```python
from build123d import *

# Parameters (mm, degrees)
BOX006_W        = 88.9
BOX006_H        = 88.9
BOX006_DEPTH    = 2438.4
SKETCH003_W     = 38.1
SKETCH003_H     = 88.9
POCKET003_DEPTH = 88.9010000032
POCKET009_DEPTH = 88.901
POCKET013_DEPTH = 38.1
SKETCH018_W     = 38.1
SKETCH018_H     = 101.6
POCKET015_DEPTH = 88.901


with BuildPart() as obj1:
    # Box006 → Box006 (new body)
    with BuildSketch(Plane(origin=(1435.1, 1435.1, 0), x_dir=(1, 0, 0), z_dir=(0, 0, 1))):
        with Locations((44.45, 44.45)):
            Rectangle(BOX006_W, BOX006_H)
    extrude(amount=BOX006_DEPTH)

    # Sketch003 → Pocket003 (cut, through all)
    with BuildSketch(Plane(origin=(1435.1, 1435.1, 0), x_dir=(1, 0, 0), z_dir=(0, -1, 0))):
        with Locations((69.85, 501.65)):
            Rectangle(SKETCH003_W, SKETCH003_H)
    extrude(amount=-POCKET003_DEPTH, mode=Mode.SUBTRACT)


with BuildPart() as pocket015:
    # Part__Mirroring: instance of obj1
    add(obj1.part.mirror(Plane(origin=(762, 0, 0), x_dir=(0, -1, 0), z_dir=(1, 0, 0))))

    # Sketch010 → Pocket009 (cut, through all)
    with BuildSketch(Plane(origin=(0, 0, 0), x_dir=(0, -1, 0), z_dir=(-1, 0, 0))):
        Polygon((-1524.003048, 2221.9412), (-1524.003048, 2438.4), (-1434.087048, 2438.4), (-1434.087048, 2189.2144524157), align=None)
    extrude(amount=-POCKET009_DEPTH, mode=Mode.SUBTRACT)

    # Sketch014 → Pocket013 (cut)
    with BuildSketch(Plane(origin=(0, 0, 0), x_dir=(0, -1, 0), z_dir=(-1, 0, 0))):
        Polygon((-1524, 2221.9412), (-1435.1, 2189.5842461737), (-1435.1, 2049.8842461737), (-1524, 2082.2412), align=None)
    extrude(amount=-POCKET013_DEPTH, mode=Mode.SUBTRACT)

    # Sketch018 → Pocket015 (cut, through all)
    with BuildSketch(Plane.YZ.offset(88.9)):
        with Locations((1504.95, 2171.7)):
            Rectangle(SKETCH018_W, SKETCH018_H)
    extrude(amount=-POCKET015_DEPTH, mode=Mode.SUBTRACT)


solid = pocket015.part
```
Check sheet for the modelled part. Datum: model origin and axes. Units: mm. A direction names the side the tool comes from. Give positions to 0.01 mm unless a question says otherwise; leave off trailing zeros. Order: outer loops, then holes, each group sorted by start corner. A loop starts at its lowest first (then second) coordinate and runs counter-clockwise, first axis right, second up. Notation, with made-up numbers: M -23.75,70 L 17.25,70 A20 ccw 17.25,97 Z; hole C 61.25,76.25 d10. An arc over 180 degrees is marked long. Answer in a Markdown table with one row per item. Add a question column.
Q1. Sectioned sample at A-A, the plane y = 1504.5. Record the boundary of the cut face in (x, z).
Q2. Thickness scan on L1, parallel to X at y = 1488, z = 2111.5; L2, parallel to Z at x = 73, y = 1502; L3, parallel to Z at x = 4, y = 1484. Record the ranges inside material, lowest first.
Q3. Access from +Z, -Z, +X, -X, +Y, -Y to the whole of each face (thin tool, end or side, straight path). Record for faces 1 (the flat face through (45, 1480, 0)), 2 (the flat face through (45, 1524, 1046)), 3 (the flat face through (38.1, 1469, 2130)), 4 (the flat face through (19, 1479, 546.1)), 5 (the flat face through (64, 1505, 2120.9)).
Q4. Gauge pin test, flat ends, axial feed: pin 1 Ø10 at (y, z) = (1499.5, 507) entering from -X; pin 2 Ø10 at (x, y) = (73, 1458.5) entering from +Z; pin 3 Ø12 at (x, y) = (71.5, 1467) entering from +Z. Record the tip position at first contact, or that the pin passes through.
Q5. Sectioned sample at B-B, the plane x = 74.5. Record the boundary of the cut face in (y, z), and give its area (3 significant figures).
Verdict:
| question | item | result |
|---|---|---|
| 1 | outline | M 0,0 L 88.9,0 L 88.9,2120.9 L 38.1,2120.9 L 38.1,2075.14 L 0,2075.14 L 0,546.1 L 38.1,546.1 L 38.1,457.2 L 0,457.2 Z |
| 2 | L1 | 38.1 to 88.9 |
| 2 | L2 | 0 to 2120.9 |
| 2 | L3 | 0 to 457.2, 546.1 to 2067.68 |
| 3 | face 1 | -Z, +X, -X, +Y, -Y |
| 3 | face 2 | +Z, -Z, +X, -X, +Y |
| 3 | face 3 | +Z, -X, -Y |
| 3 | face 4 | -X, +Y, -Y |
| 3 | face 5 | +Z, +X, -X, +Y |
| 4 | pin 1 | x = 38.1 |
| 4 | pin 2 | z = 2199.92 |
| 4 | pin 3 | z = 2203.38 |
| 5 | outline | M 1435.1,0 L 1524,0 L 1524,2120.9 L 1485.9,2120.9 L 1485.9,2208.07 L 1435.1,2189.58 Z |
| 5 | area | 193,000 mm² |
